CAD build for the part. Positions are in the model's coordinates, mm. Give positions to 0.01 mm unless a question says otherwise; leave off trailing zeros. Order: outer loops, then holes, each group sorted by start corner. A loop starts at its lowest first (then second) coordinate and runs counter-clockwise, first axis right, second up. Notation, with made-up numbers: (69.25, 87) -> (105.25, 87) arc R26 ccw to (105.25, 118) -> close; hole circle Ø9 at (-32, 23.25). An arc over 180 degrees is marked (long way). Answer as CSV lines item,"result".
```python
from build123d import *

# Parameters (mm, degrees)
SKETCH_1_R          = 28
EXTRUDE_1_DEPTH     = 1
SKETCH_2_R          = 4
CUT_EXTRUDE_1_DEPTH = 1
CUT_EXTRUDE_2_REACH = 41.611
SKETCH_3_R          = 1.5
CUT_EXTRUDE_3_REACH = 41.611
SKETCH_4_R          = 6


with BuildPart() as part:
    # 草图1 → 凸台-拉伸1 (new body)
    with BuildSketch(Plane.XY):
        Circle(SKETCH_1_R)
    extrude(amount=EXTRUDE_1_DEPTH)

    # 草图2 → 切除-拉伸1 (cut)
    with BuildSketch(Plane.XY.offset(1)):
        Circle(SKETCH_2_R)
    extrude(amount=-CUT_EXTRUDE_1_DEPTH, mode=Mode.SUBTRACT)

    # 草图3 → 切除-拉伸2 (cut, up to next)
    with BuildSketch(Plane.XY.offset(1), mode=Mode.PRIVATE) as cut_extrude_2_sk1:
        with Locations((0, 12.5)):
            Circle(SKETCH_3_R)
    cut_extrude_2_tool1 = extrude(cut_extrude_2_sk1.sketch, amount=-CUT_EXTRUDE_2_REACH, mode=Mode.PRIVATE) & part.part
    # 草图3 → 切除-拉伸2 (cut, up to next)
    with BuildSketch(Plane.XY.offset(1), mode=Mode.PRIVATE) as cut_extrude_2_sk2:
        with Locations((0, -12.5)):
            Circle(SKETCH_3_R)
    cut_extrude_2_tool2 = extrude(cut_extrude_2_sk2.sketch, amount=-CUT_EXTRUDE_2_REACH, mode=Mode.PRIVATE) & part.part
    # 草图3 → 切除-拉伸2 (cut, up to next)
    with BuildSketch(Plane.XY.offset(1), mode=Mode.PRIVATE) as cut_extrude_2_sk3:
        with Locations((12.5, 0)):
            Circle(SKETCH_3_R)
    cut_extrude_2_tool3 = extrude(cut_extrude_2_sk3.sketch, amount=-CUT_EXTRUDE_2_REACH, mode=Mode.PRIVATE) & part.part
    # 草图3 → 切除-拉伸2 (cut, up to next)
    with BuildSketch(Plane.XY.offset(1), mode=Mode.PRIVATE) as cut_extrude_2_sk4:
        with Locations((-12.5, 0)):
            Circle(SKETCH_3_R)
    cut_extrude_2_tool4 = extrude(cut_extrude_2_sk4.sketch, amount=-CUT_EXTRUDE_2_REACH, mode=Mode.PRIVATE) & part.part
    add(cut_extrude_2_tool1.solids().sort_by_distance((0, 12.5, 1))[0], mode=Mode.SUBTRACT)
    add(cut_extrude_2_tool2.solids().sort_by_distance((0, -12.5, 1))[0], mode=Mode.SUBTRACT)
    add(cut_extrude_2_tool3.solids().sort_by_distance((12.5, 0, 1))[0], mode=Mode.SUBTRACT)
    add(cut_extrude_2_tool4.solids().sort_by_distance((-12.5, 0, 1))[0], mode=Mode.SUBTRACT)

    # 草图4 → 切除-拉伸3 (cut, up to next)
    with BuildSketch(Plane.XY.offset(1), mode=Mode.PRIVATE) as cut_extrude_3_sk1:
        with Locations((11.313708499, -11.313708499)):
            Circle(SKETCH_4_R)
    cut_extrude_3_tool1 = extrude(cut_extrude_3_sk1.sketch, amount=-CUT_EXTRUDE_3_REACH, mode=Mode.PRIVATE) & part.part
    # 草图4 → 切除-拉伸3 (cut, up to next)
    with BuildSketch(Plane.XY.offset(1), mode=Mode.PRIVATE) as cut_extrude_3_sk2:
        with Locations((-11.313708499, -11.313708499)):
            Circle(SKETCH_4_R)
    cut_extrude_3_tool2 = extrude(cut_extrude_3_sk2.sketch, amount=-CUT_EXTRUDE_3_REACH, mode=Mode.PRIVATE) & part.part
    # 草图4 → 切除-拉伸3 (cut, up to next)
    with BuildSketch(Plane.XY.offset(1), mode=Mode.PRIVATE) as cut_extrude_3_sk3:
        with Locations((-11.313708499, 11.313708499)):
            Circle(SKETCH_4_R)
    cut_extrude_3_tool3 = extrude(cut_extrude_3_sk3.sketch, amount=-CUT_EXTRUDE_3_REACH, mode=Mode.PRIVATE) & part.part
    # 草图4 → 切除-拉伸3 (cut, up to next)
    with BuildSketch(Plane.XY.offset(1), mode=Mode.PRIVATE) as cut_extrude_3_sk4:
        with Locations((11.313708499, 11.313708499)):
            Circle(SKETCH_4_R)
    cut_extrude_3_tool4 = extrude(cut_extrude_3_sk4.sketch, amount=-CUT_EXTRUDE_3_REACH, mode=Mode.PRIVATE) & part.part
    add(cut_extrude_3_tool1.solids().sort_by_distance((11.313708, -11.313708, 1))[0], mode=Mode.SUBTRACT)
    add(cut_extrude_3_tool2.solids().sort_by_distance((-11.313708, -11.313708, 1))[0], mode=Mode.SUBTRACT)
    add(cut_extrude_3_tool3.solids().sort_by_distance((-11.313708, 11.313708, 1))[0], mode=Mode.SUBTRACT)
    add(cut_extrude_3_tool4.solids().sort_by_distance((11.313708, 11.313708, 1))[0], mode=Mode.SUBTRACT)


solid = part.part
```
1) Band-saw the part on C-C, the plane y = 7. Write the cut outline in (x, z).
Data:
outline,"(-27.11, 0) -> (-15.48, 0) -> (-15.48, 1) -> (-27.11, 1) -> close; (-7.14, 0) -> (7.14, 0) -> (7.14, 1) -> (-7.14, 1) -> close; (15.48, 0) -> (27.11, 0) -> (27.11, 1) -> (15.48, 1) -> close"
2) Wall check: line 1 along Y through (x, z) = (0, 0.65); line 2 along X through (y, z) = (-6, 0.35); line 3 along Y through (x, z) = (8, 0.4). Give the ranges that are in metal, low to high. Write a range as [from, to].
Data:
line 1,"y = [-28, -14], [-11, -4], [4, 11], [14, 28]"
line 2,"x = [-27.35, -14.1], [-8.53, 8.53], [14.1, 27.35]"
line 3,"y = [-26.83, -16.32], [-6.31, 6.31], [16.32, 26.83]"
3) Pin check, flat tip, straight feed: P1, Ø5, axis at x = 1.5, y = 16, coming from the -Z side. Stop position of the tip, or through.
Data:
P1,"stops at z = 0"
4) Band-saw the part on D-D, the plane z = 0.3. Give the number of separate pieces and of enclosed holes in the cut face, then the cut area to 3 significant figures.
Data:
separate pieces,"1"
enclosed holes,"9"
area,"1,930 mm2"
5) Pull direction X, two halves, no side cores. Call faces 1 (the cylindrical face through (17.037, 13.116, 0.507)), 2 (the flat face through (6, 0, 1)), 3 (the cylindrical face through (25.865, -10.724, 0.493)), 4 (the cylindrical face through (16.856, -13.612, 0.507)): pulls with the +X half, pulls with the -X half, needs draft (parallel to the pull), parting line crosses it, or undercut.
Data:
face 1,"undercut"
face 2,"needs draft"
face 3,"parting line crosses it"
face 4,"undercut"
6) Band-saw the part on A-A, the plane x = 0. Write the cut outline in (y, z), then the cut area to 3 significant figures.
Data:
outline,"(-28, 0) -> (-14, 0) -> (-14, 1) -> (-28, 1) -> close; (-11, 0) -> (-4, 0) -> (-4, 1) -> (-11, 1) -> close; (4, 0) -> (11, 0) -> (11, 1) -> (4, 1) -> close; (14, 0) -> (28, 0) -> (28, 1) -> (14, 1) -> close"
area,"42.0 mm2"
